The model under review builds one solid part; all positions refer to its coordinate system, in mm. A direction names the side the tool comes from. Coordinates: 2 decimals unless noted, no trailing zeros. Order: outer loops, then holes, each group sorted by start corner. A loop starts at its lowest first (then second) coordinate and runs counter-clockwise, first axis right, second up.
from build123d import *

# Parameters (mm, degrees)
SKETCH1_W                                        = 100
SKETCH1_H                                        = 12.7
BOSS_EXTRUDE1_DEPTH                              = 55
M4_CLEARANCE_HOLE1_D                             = 4.5
CBORE_FOR_1_4_SOCKET_HEAD_CAP_SCREW1_D           = 6.7564
CBORE_FOR_1_4_SOCKET_HEAD_CAP_SCREW1_CBORE_D     = 11.1125
CBORE_FOR_1_4_SOCKET_HEAD_CAP_SCREW1_CBORE_DEPTH = 6.35


with BuildPart() as part:
    # Sketch1 → Boss-Extrude1 (new, symmetric)
    with BuildSketch(Plane.XY):
        Rectangle(SKETCH1_W, SKETCH1_H)
    extrude(amount=BOSS_EXTRUDE1_DEPTH, both=True)

    # M4 Clearance Hole1 (through all)
    with Locations(Plane(origin=(0, 6.35, 0), x_dir=(1, 0, 0), z_dir=(0, 1, 0))):
        with Locations((14.5, -47), (-14.5, -47), (-14.5, 47), (14.5, 47)):
            Hole(M4_CLEARANCE_HOLE1_D / 2)

    # CBORE for 1/4 Socket Head Cap Screw1 (through all)
    with Locations(Plane(origin=(0, -6.35, 0), x_dir=(-1, 0, 0), z_dir=(0, -1, 0))):
        with Locations((30.000007891, 1.671e-06), (-29.999992109, 1.671e-06)):
            CounterBoreHole(CBORE_FOR_1_4_SOCKET_HEAD_CAP_SCREW1_D / 2, CBORE_FOR_1_4_SOCKET_HEAD_CAP_SCREW1_CBORE_D / 2, CBORE_FOR_1_4_SOCKET_HEAD_CAP_SCREW1_CBORE_DEPTH)


solid = part.part
(1) Consider section A-A (x = -14.5). Give the boundary of the cut face in (y, z), then the cut area to 3 significant figures.
(2) Consider section B-B (z = -47). Give the boundary of the cut face in (x, y).
(3) Insertion check: pin 1 Ø9 at (x, z) = (-30, 0) entering from -Y. The pin has a flat end and moves straight along its axis. Give the tip position at first contact, or say it passes through.
(4) Tool access review of faces 1 (the face through (-26.879, 3.219, 1.294)), 2 (the face through (24.7, -3.22, -1.67)): name each direction out of +Z, -Z, +X, -X, +Y, -Y from which nothing blocks a thin tool from reaching the whole face with its end or side.
(5) Wall thickness on line 1 (Z direction, x = 14.5, y = -0.5); line 2 (X direction, y = 0, z = -47); line 3 (X direction, y = 0.75, z = -46): over which ranges is each line inside the solid? List them lowest first.
(6) The part is to be moulded in two halves that separate along Z. For faces 3 (the face through (-1, 0, 55)), 4 (the face through (-50, 0, 1)), 5 (the face through (-35.13, -3.22, 2.13)), say which applies: +Z half, -Z half, draft (parallel to the pull), parting line (faces both ways), or undercut.
(7) Consider section C-C (x = 29.5). Give the boundary of the cut face in (y, z).
Findings:
1. outline: (-6.35, -55) - (6.35, -55) - (6.35, -49.25) - (-6.35, -49.25) - close; (-6.35, -44.75) - (6.35, -44.75) - (6.35, 44.75) - (-6.35, 44.75) - close; (-6.35, 49.25) - (6.35, 49.25) - (6.35, 55) - (-6.35, 55) - close
1. area: 1,280 mm2
2. outline: (-50, -6.35) - (-16.75, -6.35) - (-16.75, 6.35) - (-50, 6.35) - close; (-12.25, -6.35) - (12.25, -6.35) - (12.25, 6.35) - (-12.25, 6.35) - close; (16.75, -6.35) - (50, -6.35) - (50, 6.35) - (16.75, 6.35) - close
3. pin 1: stops at y = 0
4. face 1: +Y, -Y
4. face 2: -Y
5. line 1: z = -55 to -49.25, -44.75 to 44.75, 49.25 to 55
5. line 2: x = -50 to -16.75, -12.25 to 12.25, 16.75 to 50
5. line 3: x = -50 to -16.52, -12.48 to 12.48, 16.52 to 50
6. face 3: +Z half
6. face 4: draft
6. face 5: undercut
7. outline: (-6.35, -55) - (6.35, -55) - (6.35, -3.34) - (0, -3.34) - (0, -5.53) - (-6.35, -5.53) - close; (-6.35, 5.53) - (0, 5.53) - (0, 3.34) - (6.35, 3.34) - (6.35, 55) - (-6.35, 55) - close
